Input: part model. Units: mm. Frame: model coordinates. Face numbers are marked on the shaded views. A direction names the side the tool comes from. Round coordinates to 2 decimals unless told otherwise and drop trailing zeros. Order: outer loops, then holes, each group sorted by start corner. A loop starts at its lowest first (then second) coordinate and runs counter-clockwise, first axis right, second up. Notation, with made-up numbers: (14.5, 51.5) -> (57.5, 51.5) arc R24 ccw to (57.5, 89.5) -> close; hole circle Ø5 at (-28.75, -24.5). An arc over 180 degrees is marked (long way). Use a Markdown table: item, result.
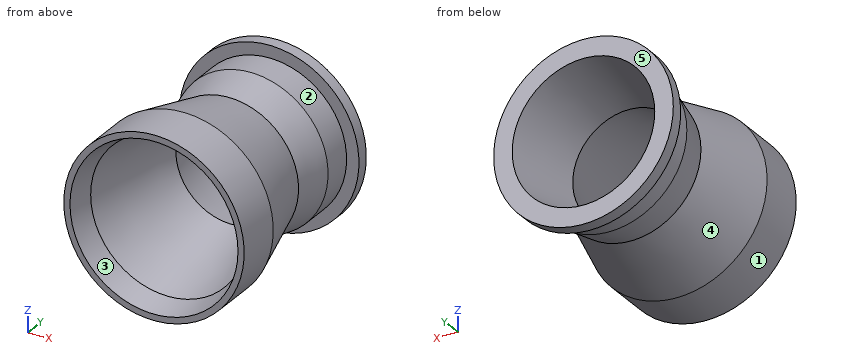
Autodesk Inventor part; units mm, degrees
ref_plane "YZ Plane" through (0, 0, 0) normal (1, 0, 0) x (0, 1, 0)
ref_plane "XZ Plane" through (0, 0, 0) normal (0, 1, 0) x (-1, 0, 0)
ref_plane "XY Plane" through (0, 0, 0) normal (0, 0, 1) x (1, 0, 0)
sketch "Sketch1" plane through (0, 0, 0) normal (0, 0, 1) x (1, 0, 0)
  line L0 (0, 25.4) -> (-28.702, 25.4) construction
  line L1 (0, 25.4) -> (-95.25, 25.4) construction
  line L2 (-95.25, 25.4) -> (-89.1588, 25.4) construction
  line L3 (-89.1588, 25.4) -> (-85.693, 23.7839) construction
  line L4 (-89.1588, 25.4) -> (-89.1588, 21.1626) construction
  line L5 (-89.1588, 0) -> (-95.25, 0)
  line L6 (-28.702, 59.6457) -> (-28.702, -91.9304) construction
  arc A0 (-28.9184, -8.4804) -> (-32.3684, -1.0818) centre (-35.052, -6.8369) ccw
  line L7 (-89.1588, 25.4) -> (-89.1588, 0)
  line L8 (-89.1588, 25.4) -> (-32.3684, -1.0818)
  line L9 (-28.9184, -8.4804) -> (-28.9392, -8.5583)
  line L10 (0, -319.0244) -> (0, 122.7573)
  line L11 (-73.152, 17.9359) -> (-28.702, 17.9359) construction
  line L12 (-89.1588, 0) -> (-92.3338, 0)
  line L13 (11.4547, -6.8369) -> (-136.2084, -6.8369) construction
  line L14 (-57.2892, -89.8271) -> (-86.36, -198.3209)
  line L15 (-92.3338, -12.7) -> (-73.2838, -12.7)
  line L16 (-73.2838, -12.7) -> (-54.421, -103.6575)
  line L17 (-92.71, -222.8555) -> (-86.36, -222.8555)
  line L18 (-86.36, -198.3209) -> (-79.786, -198.3209)
  line L19 (-92.71, -172.9504) -> (-71.7053, -94.5599)
  line L20 (-92.3338, -25.4) -> (-79.6338, -25.4)
  line L21 (-79.6338, -25.4) -> (-79.6338, -57.15)
  line L22 (-79.6338, -57.15) -> (-71.7053, -94.5599)
  line L23 (-92.3338, 0) -> (-92.3338, -25.4)
  line L24 (-92.71, -172.9504) -> (-92.71, -222.8555)
  line L25 (-86.3902, -25.4) -> (-86.3902, -31.3436)
  line L26 (-86.3902, -31.3436) -> (-92.3338, -31.3436)
  line L27 (-92.3338, -31.3436) -> (-92.3338, -56.7436)
  line L28 (-92.3338, -56.7436) -> (-79.6338, -56.7436)
  line L29 (-73.152, 17.9359) -> (-32.3684, -1.0818)
  line L30 (-73.152, 17.9359) -> (-50.7653, -90.0141)
  line L31 (-50.7653, -90.0141) -> (-28.9184, -8.4804)
  line L32 (-52.4654, -96.3589) -> (-28.9184, -8.4804)
  line L33 (-86.36, -222.8555) -> (-28.9184, -8.4804)
  point P0 (0, 0)
  point P1 (-95.25, -255.9127)
  point P2 (-88.7095, 22.4389)
  dimension "d0" = 28.702
  dimension "d3" = 25
  dimension "d5" = 25.4
  dimension "d6" = 25.4
  dimension "d8" = 12.7
  dimension "d34" = 15
  dimension "d37" = 44.45
  dimension "d46" = 19.05
  dimension "d47" = 12.7
  dimension "d50" = 86.36
  dimension "d53" = 12.7
  dimension "d55" = 12.7
  dimension "d56" = 31.75
  dimension "d58" = 0.25
  dimension "d60" = 12.7
  dimension "d61" = 25.4
  dimension "d62" = 5.9436
  dimension "d63" = 5.9436
  dimension "d64" = 3.175
  dimension "d65" = 6.35
  dimension "d67" = 6.35
  dimension "d68" = 107.95
  dimension "d69" = 6.35
  dimension "d70" = 6.35
revolve "Revolution2" add sketch "Sketch1" angle 360 about axis through (0, -10, 0) along (0, 1, 0) contours L15 L16 L14 L18 L33 L17 L24 L19 L22 L21 L20 L23
properties part number "aluminum" material "Aluminum 6061"
1) Cut plane A-A on x = 0. Return loops of the section in (y, z).
Answer key:
| item | result |
|---|---|
| outline | (-222.86, -92.71) -> (-172.95, -92.71) -> (-94.56, -71.71) -> (-57.15, -79.63) -> (-25.4, -79.63) -> (-25.4, -92.33) -> (-12.7, -92.33) -> (-12.7, -73.28) -> (-89.83, -57.29) -> (-198.32, -86.36) -> (-198.32, -79.79) -> (-222.86, -86.36) -> close; (-222.86, 86.36) -> (-198.32, 79.79) -> (-198.32, 86.36) -> (-89.83, 57.29) -> (-12.7, 73.28) -> (-12.7, 92.33) -> (-25.4, 92.33) -> (-25.4, 79.63) -> (-57.15, 79.63) -> (-94.56, 71.71) -> (-172.95, 92.71) -> (-222.86, 92.71) -> close |
2) Draft query along X for the marked faces 3, 4 and 5. Return one class per face: released by +X, released by -X, zero draft, split by the parting line, or undercut.
Answer key:
| item | result |
|---|---|
| face 3 | undercut |
| face 4 | split by the parting line |
| face 5 | zero draft |
3) Cut plane D-D on y = -208. Return loops of the section in (x, z), and give its area (3 significant figures).
Answer key:
| item | result |
|---|---|
| outline | circle Ø185.42 at (0, 0); hole circle Ø164.76 at (0, 0) |
| area | 5,680 mm^2 |
4) Set-up query: the marked faces 1 and 2. Return all of +Z, -Z, +X, -X, +Y, -Y with unobstructed straight access to the full face (end or side cutting, diameter ignored); none if empty.
Answer key:
| item | result |
|---|---|
| face 1 | +Y, -Y |
| face 2 | none |
5) Cut plane B-B on z = 0. Return loops of the section in (x, y).
Answer key:
| item | result |
|---|---|
| outline | (-92.71, -222.86) -> (-86.36, -222.86) -> (-79.79, -198.32) -> (-86.36, -198.32) -> (-57.29, -89.83) -> (-73.28, -12.7) -> (-92.33, -12.7) -> (-92.33, -25.4) -> (-79.63, -25.4) -> (-79.63, -57.15) -> (-71.71, -94.56) -> (-92.71, -172.95) -> close; (57.29, -89.83) -> (86.36, -198.32) -> (79.79, -198.32) -> (86.36, -222.86) -> (92.71, -222.86) -> (92.71, -172.95) -> (71.71, -94.56) -> (79.63, -57.15) -> (79.63, -25.4) -> (92.33, -25.4) -> (92.33, -12.7) -> (73.28, -12.7) -> close |
6) Ray query, probe 1 along Z at (x, y) = (-54.5, -34); probe 2 along X at (y, z) = (-125, 42); probe 3 along X at (y, z) = (-55, 38). Return the intervals inside material, ascending.
Answer key:
| item | result |
|---|---|
| probe 1 | z = -58.06 to -42.1, 42.1 to 58.06 |
| probe 2 | x = -67.93 to -51.83, 51.83 to 67.93 |
| probe 3 | x = -69.98 to -52.13, 52.13 to 69.98 |
7) Contact query for flat-ended pins moving along their axis: P1, Ø1, axis at y = -133, z = -47.5, coming from the +X side; P2, Ø2, axis at y = -72, z = 24, coming from the +X side; P3, Ø6, axis at y = -85.5, z = 63.5, coming from the -X side. Output: stop coordinate, or through.
Answer key:
| item | result |
|---|---|
| P1 | stops at x = 67.24 |
| P2 | stops at x = 73.02 |
| P3 | stops at x = -42.1 |
8) Cut plane C-C on y = -149.5. Return loops of the section in (x, z), and give its area (3 significant figures).
Answer key:
| item | result |
|---|---|
| outline | circle Ø172.85 at (0, 0); hole circle Ø146.56 at (0, 0) |
| area | 6,600 mm^2 |
